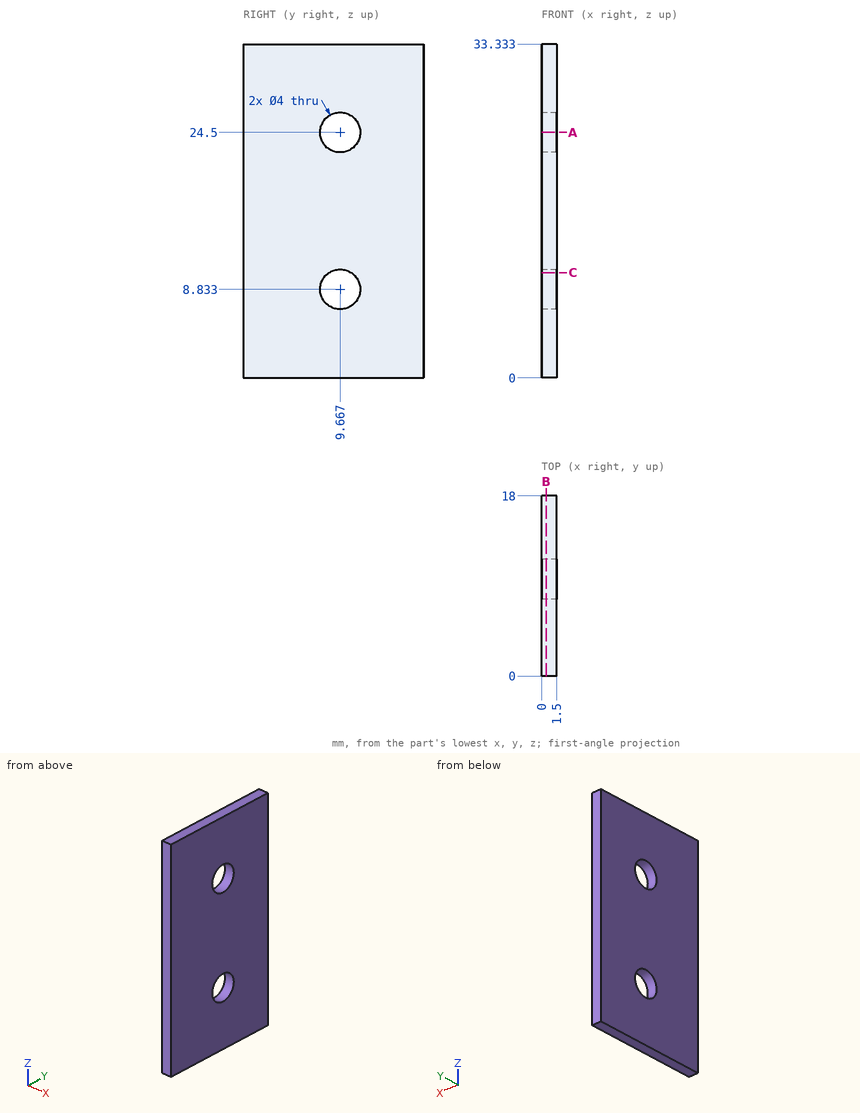
Answer from the drawing. Dimensions are ordinates in mm from the lowest x, y and z of the part. Give positions to 0.01 mm unless a question says otherwise; leave off trailing zeros. Loops run counter-clockwise (first coordinate to the right, second up) from the corner with the lowest first, then second, coordinate; pieces in that order, holes last.
Item 1: The part is cut by section B-B (x = 0.45). Write down the section's boundary in (y, z).
Item 2: Find the intervals of material crossed by line 1 along Z through (x, y) = (0.65, 10) (1 decimal); line 2 along Y through (x, z) = (0.95, 9); line 3 along Z through (x, y) = (1.45, 9) (1 decimal), in increasing order.
Item 3: The part is cut by section C-C (z = 10.5). Write down the section's boundary in (x, y).
Item 4: The part is cut by section A-A (z = 24.5). Write down the section's boundary in (x, y), and give its area (3 significant figures).
Taken from the geometry:
1. outline: (0, 0) - (18, 0) - (18, 33.33) - (0, 33.33) - close; hole circle Ø4 at (9.67, 8.83); hole circle Ø4 at (9.67, 24.5)
2. line 1: z = 0 to 6.9, 10.8 to 22.5, 26.5 to 33.3
2. line 2: y = 0 to 7.67, 11.66 to 18
2. line 3: z = 0 to 6.9, 10.7 to 22.6, 26.4 to 33.3
3. outline: (0, 0) - (1.5, 0) - (1.5, 8.56) - (0, 8.56) - close; (0, 10.77) - (1.5, 10.77) - (1.5, 18) - (0, 18) - close
4. outline: (0, 0) - (1.5, 0) - (1.5, 7.67) - (0, 7.67) - close; (0, 11.67) - (1.5, 11.67) - (1.5, 18) - (0, 18) - close
4. area: 21.0 mm2
